Could you check a few things on this model? Use its own coordinates, in mm. Coordinates: 2 decimals unless noted, no trailing zeros. Loops run counter-clockwise (first coordinate to the right, second up) from the corner with the lowest first, then second, coordinate; pieces in that order, holes last.
from build123d import *

# Parameters (mm, degrees)
SKETCH1_R           = 177
SKETCH1_R_2         = 1.6
SKETCH1_R_3         = 2.2479
SKETCH1_R_4         = 2.000000064
SKETCH1_R_5         = 1.3
SKETCH1_R_6         = 1.29999994
SKETCH1_W           = 6.15
SKETCH1_H           = 6.15
SKETCH1_W_2         = 30
SKETCH1_H_2         = 80
SKETCH1_W_3         = 6.35
SKETCH1_H_3         = 3.175
BOSS_EXTRUDE1_DEPTH = 4.7625


with BuildPart() as part:
    # Sketch1 → Boss-Extrude1 (new body)
    with BuildSketch(Plane(origin=(0, 0, 0), x_dir=(1, 0, 0), z_dir=(0, 1, 0))):
        with Locations(Location((0, 0, 0), (0, 0, 90))):
            Circle(SKETCH1_R)
        with Locations(Location((-150.65, 25.4, 0), (0, 0, 90))):
            Circle(SKETCH1_R_2, mode=Mode.SUBTRACT)
        with Locations(Location((-150.65, -25.4, 0), (0, 0, 90))):
            Circle(SKETCH1_R_2, mode=Mode.SUBTRACT)
        with Locations(Location((150.65, 25.4, 0), (0, 0, 90))):
            Circle(SKETCH1_R_2, mode=Mode.SUBTRACT)
        with Locations(Location((150.65, -25.4, 0), (0, 0, 90))):
            Circle(SKETCH1_R_2, mode=Mode.SUBTRACT)
        with Locations(Location((-107.95, 25.4, 0), (0, 0, 90))):
            Circle(SKETCH1_R_2, mode=Mode.SUBTRACT)
        with Locations(Location((-107.95, -25.4, 0), (0, 0, 90))):
            Circle(SKETCH1_R_2, mode=Mode.SUBTRACT)
        with Locations(Location((107.95, 25.4, 0), (0, 0, 90))):
            Circle(SKETCH1_R_2, mode=Mode.SUBTRACT)
        with Locations(Location((107.95, -25.4, 0), (0, 0, 90))):
            Circle(SKETCH1_R_2, mode=Mode.SUBTRACT)
        with Locations(Location((-53.7, 107.95, 0), (0, 0, 90))):
            Circle(SKETCH1_R_2, mode=Mode.SUBTRACT)
        with Locations(Location((38.8, 107.95, 0), (0, 0, 90))):
            Circle(SKETCH1_R_2, mode=Mode.SUBTRACT)
        with Locations(Location((-53.7, 29.45, 0), (0, 0, 90))):
            Circle(SKETCH1_R_2, mode=Mode.SUBTRACT)
        with Locations(Location((38.8, 29.45, 0), (0, 0, 90))):
            Circle(SKETCH1_R_2, mode=Mode.SUBTRACT)
        with Locations(Location((-101.6, -101.6, 0), (0, 0, 90))):
            Circle(SKETCH1_R_3, mode=Mode.SUBTRACT)
        with Locations(Location((101.6, -101.6, 0), (0, 0, 90))):
            Circle(SKETCH1_R_3, mode=Mode.SUBTRACT)
        with Locations(Location((-101.6, 101.6, 0), (0, 0, 90))):
            Circle(SKETCH1_R_3, mode=Mode.SUBTRACT)
        with Locations(Location((101.6, 101.6, 0), (0, 0, 90))):
            Circle(SKETCH1_R_3, mode=Mode.SUBTRACT)
        with Locations(Location((-20, -142.687006289, 0), (0, 0, 90))):
            Circle(SKETCH1_R_4, mode=Mode.SUBTRACT)
        with Locations(Location((20, -142.687006289, 0), (0, 0, 90))):
            Circle(SKETCH1_R_4, mode=Mode.SUBTRACT)
        with Locations(Location((-20, 151.719279026, 0), (0, 0, 90))):
            Circle(SKETCH1_R_4, mode=Mode.SUBTRACT)
        with Locations(Location((20, 151.719279026, 0), (0, 0, 90))):
            Circle(SKETCH1_R_4, mode=Mode.SUBTRACT)
        with Locations(Location((-10.125, -171.45, 0), (0, 0, 90))):
            Circle(SKETCH1_R_5, mode=Mode.SUBTRACT)
        with Locations(Location((10.125, -171.45, 0), (0, 0, 90))):
            Circle(SKETCH1_R_6, mode=Mode.SUBTRACT)
        with Locations(Location((171.45, -10.125, 0), (0, 0, 90))):
            Circle(SKETCH1_R_5, mode=Mode.SUBTRACT)
        with Locations(Location((171.45, 10.125, 0), (0, 0, 90))):
            Circle(SKETCH1_R_5, mode=Mode.SUBTRACT)
        with Locations(Location((-171.45, -10.125, 0), (0, 0, 90))):
            Circle(SKETCH1_R_5, mode=Mode.SUBTRACT)
        with Locations(Location((-171.45, 10.125, 0), (0, 0, 90))):
            Circle(SKETCH1_R_5, mode=Mode.SUBTRACT)
        with Locations(Location((-63.76, 13.473999986, 0), (0, 0, 90))):
            Circle(SKETCH1_R_2, mode=Mode.SUBTRACT)
        with Locations(Location((-63.76, -13.450000014, 0), (0, 0, 90))):
            Circle(SKETCH1_R_2, mode=Mode.SUBTRACT)
        with Locations(Location((-21.85, 13.473999986, 0), (0, 0, 90))):
            Circle(SKETCH1_R_2, mode=Mode.SUBTRACT)
        with Locations(Location((-21.85, -13.450000014, 0), (0, 0, 90))):
            Circle(SKETCH1_R_2, mode=Mode.SUBTRACT)
        with Locations(Location((63.76, -13.450000014, 0), (0, 0, 90))):
            Circle(SKETCH1_R_2, mode=Mode.SUBTRACT)
        with Locations(Location((21.85, -13.450000014, 0), (0, 0, 90))):
            Circle(SKETCH1_R_2, mode=Mode.SUBTRACT)
        with Locations(Location((21.85, 13.473999986, 0), (0, 0, 90))):
            Circle(SKETCH1_R_2, mode=Mode.SUBTRACT)
        with Locations(Location((63.76, 13.473999986, 0), (0, 0, 90))):
            Circle(SKETCH1_R_2, mode=Mode.SUBTRACT)
        with Locations((171.45, 4.26)):
            Rectangle(SKETCH1_W, SKETCH1_H, mode=Mode.SUBTRACT)
        with Locations((-129.3, 0)):
            Rectangle(SKETCH1_W_2, SKETCH1_H_2, mode=Mode.SUBTRACT)
        with Locations((129.3, 0)):
            Rectangle(SKETCH1_W_2, SKETCH1_H_2, mode=Mode.SUBTRACT)
        with Locations((4.26, -171.45)):
            Rectangle(SKETCH1_W, SKETCH1_H, mode=Mode.SUBTRACT)
        with Locations((-171.45, 4.26)):
            Rectangle(SKETCH1_W, SKETCH1_H, mode=Mode.SUBTRACT)
        with Locations((-18.119952608, 164.452014647)):
            Rectangle(SKETCH1_W_3, SKETCH1_H_3, mode=Mode.SUBTRACT)
        with Locations((-30.819952608, 164.452014647)):
            Rectangle(SKETCH1_W_3, SKETCH1_H_3, mode=Mode.SUBTRACT)
        with Locations((-5.419952608, 164.452014647)):
            Rectangle(SKETCH1_W_3, SKETCH1_H_3, mode=Mode.SUBTRACT)
        with Locations((7.280047392, 164.452014647)):
            Rectangle(SKETCH1_W_3, SKETCH1_H_3, mode=Mode.SUBTRACT)
        with Locations((19.980047392, 164.452014647)):
            Rectangle(SKETCH1_W_3, SKETCH1_H_3, mode=Mode.SUBTRACT)
        with Locations((32.680047392, 164.452014647)):
            Rectangle(SKETCH1_W_3, SKETCH1_H_3, mode=Mode.SUBTRACT)
    extrude(amount=BOSS_EXTRUDE1_DEPTH)


solid = part.part
1) Imagine slicing it at D-D on x = 75.5. List the corners of the cut face in (y, z) for me, plus the area to 3 significant figures.
2) Imagine slicing it at A-A on x = 135.5. List the corners of the cut face in (y, z) for me, plus the area to 3 significant figures.
3) If I drill on L1, parallel to Z at x = 38.8, y = 3.4 (3 decimals); L2, parallel to X at y = 1.8, z = -29.45; L3, parallel to Z at x = 20, y = 2.15, over which ranges is the centre line in solid material (lowest first)?
4) Imagine slicing it at C-C on y = 2.95. State how many separate pieces and enclosed holes the cut face has, plus the area to 3 significant figures.
5) We'd pull the mould along X, two halves only. Please class faces 1 (the cylindrical face through (172.79, 2.35, 38.37)), 2 (the flat face through (-2, 0, 2)): released by +X, released by -X, zero draft, split by the parting line, or undercut.
6) Will these pins go through, and if not, where does the flat tip stop? pin 1 (1.9 mm diameter, centred on x = -107.95, z = -25.4, fed in from -Y); pin 2 (4 mm diameter, centred on x = -10.125, z = 171.45, fed in from -Y); pin 3 (2.5 mm diameter, centred on y = 1, z = -164, fed in from +X); pin 4 (2.5 mm diameter, centred on x = -19.5, y = 2, fed in from -Z).
7) Imagine slicing it at B-B on z = -60.5. List the corners of the cut face in (x, y) for me, plus the area to 3 significant figures.
Solved:
1. outline: (0, -160.09) - (4.76, -160.09) - (4.76, 160.09) - (0, 160.09) - close
1. area: 1,520 mm2
2. outline: (0, -113.88) - (4.76, -113.88) - (4.76, -40) - (0, -40) - close; (0, 40) - (4.76, 40) - (4.76, 113.88) - (0, 113.88) - close
2. area: 704 mm2
3. L1: z = -172.695 to -109.55, -106.35 to -31.05, -27.85 to 172.695
3. L2: x = -174.53 to -144.3, -114.3 to -55.3, -52.1 to 37.2, 40.4 to 114.3, 144.3 to 174.53
3. L3: z = -175.87 to -166.04, -162.86 to -153.72, -149.72 to 140.69, 144.69 to 175.87
4. separate pieces: 1
4. enclosed holes: 45
4. area: 93,100 mm2
5. face 1: split by the parting line
5. face 2: zero draft
6. pin 1: passes through
6. pin 2: stops at y = 0
6. pin 3: stops at x = 69.58
6. pin 4: stops at z = -176.06
7. outline: (-166.34, 0) - (166.34, 0) - (166.34, 4.76) - (-166.34, 4.76) - close
7. area: 1,580 mm2
